Could you check a few things on this model? Use its own coordinates, in mm. Face numbers are marked on the shaded views. A direction names the side the tool comes from. Coordinates: 2 decimals unless noted, no trailing zeros. Order: outer loops, then holes, each group sorted by start corner. A loop starts at its lowest first (then second) coordinate and runs counter-clockwise, first axis right, second up. Notation, with made-up numbers: (-10.75, 68.25) -> (35.25, 68.25) arc R21 cw to (35.25, 94.25) -> close; hole circle Ø4 at (10, 0). An arc over 180 degrees is marked (long way). Put each result on its own line as item: value. Start each with the question number.
Q1. If we section it at B-B (z = -9.5): Please give me the cut outline in (x, y).
Q2. If we section it at C-C (x = -8): Please give me the cut outline in (y, z).
Q3. We'd pull the mould along Y, two halves only. Please class the marked faces 1, 2 and 3: +Y half, -Y half, draft (parallel to the pull), parting line (faces both ways), or undercut.
Q4. If we section it at D-D (y = -8): Please give me the cut outline in (x, z).
Q5. Please list where these lines run through material, in increasing order: line 1 along X through (y, z) = (4, -1); line 2 along Y through (x, z) = (22, -1.5); line 3 along Y through (x, z) = (-10, 0.75).
Q6. For the marked faces 4 and 5, which set-ups out of +Z, -Z, +X, -X, +Y, -Y let a thin tool reach every point of the face, with its end or its side?
Q7. If we section it at A-A (z = -3): Count the separate pieces of the cut face and the enclosed holes in it, and give its area (3 significant figures).
Q8. Will these pins go through, and if not, where does the flat tip stop? pin 1 (3.5 mm diameter, centred on x = -24.48, y = -11.95, fed in from +Z); pin 2 (1 mm diameter, centred on y = -2.5, z = -7.5, fed in from -X); pin 3 (4.5 mm diameter, centred on x = 22.12, y = -11.95, fed in from -Z); pin 4 (3 mm diameter, centred on x = 20, y = 3, fed in from -Z).
from build123d import *

# Parameters (mm, degrees)
CROQUIS2_R                = 2.4
CROQUIS2_R_2              = 1.45
SALIENTE_EXTRUIR2_DEPTH   = 12.3
SALIENTE_EXTRUIR2_2_DEPTH = 12.3
CROQUIS2_R_3              = 2.2627417
SALIENTE_EXTRUIR2_3_DEPTH = 12.3
CROQUIS2_R_4              = 1.304870774
SALIENTE_EXTRUIR2_4_DEPTH = 12.3
CROQUIS4_W                = 36.3
CROQUIS4_H                = 63.7
CROQUIS4_W_2              = 32.3
CROQUIS4_H_2              = 59.7
SALIENTE_EXTRUIR4_DEPTH   = 8.9
CROQUIS5_W                = 36.3
CROQUIS5_H                = 63.7
SALIENTE_EXTRUIR5_DEPTH   = 2
REDONDEO1_R               = 1
CROQUIS6_W                = 0.952491513
CROQUIS6_H                = 11.029714725
CORTAR_EXTRUIR1_DEPTH     = 1
REDONDEO2_R               = 1
CROQUIS7_R                = 1.45
CROQUIS7_R_2              = 1.304870774
CORTAR_EXTRUIR2_DEPTH     = 42.540563821
CROQUIS8_R                = 2.75
CORTAR_EXTRUIR3_DEPTH     = 1
CROQUIS9_R                = 3.250192478
CORTAR_EXTRUIR4_DEPTH     = 41.895212954
CROQUIS10_W               = 30.589236147
CROQUIS10_H               = 22.63620754
CROQUIS10_W_2             = 28.589236147
CROQUIS10_H_2             = 20.63620754
SALIENTE_EXTRUIR6_DEPTH   = 2.5


with BuildPart() as part:
    # Croquis2 → Saliente-Extruir2 (new body)
    with BuildSketch(Plane(origin=(-1.363345475, 4.236097797, 1), x_dir=(0, 1, 0), z_dir=(0, 0, 1))):
        with Locations(Location((-16.185020115, 23.120880637, 0), (0, 0, 270))):
            Circle(CROQUIS2_R)
        with Locations(Location((-16.185020115, 23.120880637, 0), (0, 0, 270))):
            Circle(CROQUIS2_R_2, mode=Mode.SUBTRACT)
    extrude(amount=-SALIENTE_EXTRUIR2_DEPTH)



with BuildPart() as body_2:
    # Croquis2 → Saliente-Extruir2 2 (new body)
    with BuildSketch(Plane(origin=(-1.363345475, 4.236097797, 1), x_dir=(0, 1, 0), z_dir=(0, 0, 1))):
        with Locations(Location((7.314979885, 23.120880637, 0), (0, 0, 270))):
            Circle(CROQUIS2_R)
        with Locations(Location((7.314979885, 23.120880637, 0), (0, 0, 270))):
            Circle(CROQUIS2_R_2, mode=Mode.SUBTRACT)
    extrude(amount=-SALIENTE_EXTRUIR2_2_DEPTH)


with BuildPart() as body_3:
    # Croquis2 → Saliente-Extruir2 3 (new body)
    with BuildSketch(Plane(origin=(-1.363345475, 4.236097797, 1), x_dir=(0, 1, 0), z_dir=(0, 0, 1))):
        with Locations(Location((7.314979885, -23.479119363, 0), (0, 0, 270))):
            Circle(CROQUIS2_R_3)
        with Locations(Location((7.314979885, -23.479119363, 0), (0, 0, 270))):
            Circle(CROQUIS2_R_2, mode=Mode.SUBTRACT)
    extrude(amount=-SALIENTE_EXTRUIR2_3_DEPTH)


with BuildPart() as body_4:
    # Croquis2 → Saliente-Extruir2 4 (new body)
    with BuildSketch(Plane(origin=(-1.363345475, 4.236097797, 1), x_dir=(0, 1, 0), z_dir=(0, 0, 1))):
        with Locations(Location((-16.185020115, -23.479119363, 0), (0, 0, 270))):
            Circle(CROQUIS2_R)
        with Locations(Location((-16.185020115, -23.479119363, 0), (0, 0, 270))):
            Circle(CROQUIS2_R_4, mode=Mode.SUBTRACT)
    extrude(amount=-SALIENTE_EXTRUIR2_4_DEPTH)


with BuildPart() as body_5:
    # Croquis4 → Saliente-Extruir4 (new body)
    with BuildSketch(Plane(origin=(-1.363345475, 4.236097797, 1), x_dir=(0, 1, 0), z_dir=(0, 0, 1))):
        with Locations((-4.435020115, -3.929119363)):
            Rectangle(CROQUIS4_W, CROQUIS4_H)
        with Locations((-4.435020115, -3.929119363)):
            Rectangle(CROQUIS4_W_2, CROQUIS4_H_2, mode=Mode.SUBTRACT)
    extrude(amount=-SALIENTE_EXTRUIR4_DEPTH)


with BuildPart() as part_1:
    add(part.part)

    add(body_2.part)  # Saliente-Extruir5 merges body 2

    add(body_3.part)  # Saliente-Extruir5 merges body 3

    add(body_4.part)  # Saliente-Extruir5 merges body 4

    add(body_5.part)  # Saliente-Extruir5 merges body 5
    # Croquis5 → Saliente-Extruir5 (add)
    with BuildSketch(Plane(origin=(-1.363345475, 4.236097797, 1), x_dir=(0, 1, 0), z_dir=(0, 0, 1))):
        with Locations((-4.435020115, -3.929119363)):
            Rectangle(CROQUIS5_W, CROQUIS5_H)
    extrude(amount=SALIENTE_EXTRUIR5_DEPTH)

    # Redondeo1
    redondeo1_edges = [part_1.edges().sort_by_distance(p)[0] for p in [
        (-29.284226112, -18.348922317, -2.45),
        (34.415773888, -18.348922317, -2.45),
        (34.415773888, 17.951077683, -2.45),
        (-29.284226112, 17.951077683, -2.45),
        (2.565773888, -18.348922317, 3),
        (34.415773888, -0.198922317, 3),
        (2.565773888, 17.951077683, 3),
        (-29.284226112, -0.198922317, 3),
    ]]
    fillet(redondeo1_edges, radius=REDONDEO1_R)

    # Croquis6 → Cortar-Extruir1 (cut)
    with BuildSketch(Plane.ZY.offset(29.284226112)):
        with Locations((-7.423754244, -0.221239115)):
            Rectangle(CROQUIS6_W, CROQUIS6_H)
    extrude(amount=-CORTAR_EXTRUIR1_DEPTH, mode=Mode.SUBTRACT)

    # Redondeo2
    redondeo2_edges = [part_1.edges().sort_by_distance(p)[0] for p in [
        (-29.284226112, -5.736096478, -7.423754243),
        (-29.284226112, 5.293618247, -7.423754243),
        (-29.284226112, -0.221239116, -6.947508487),
    ]]
    fillet(redondeo2_edges, radius=REDONDEO2_R - 0.0001)  # a hair under: the kernel refuses the full size

    # Croquis7 → Cortar-Extruir2 (cut, through all)
    with BuildSketch(Plane(origin=(0, 0, -11.3), x_dir=(-1, 0, 0), z_dir=(0, 0, -1))):
        with Locations(Location((24.484226112, 11.551077683, 0), (0, 0, 180))):
            Circle(CROQUIS7_R)
        with Locations(Location((24.484226112, -11.948922317, 0), (0, 0, 180))):
            Circle(CROQUIS7_R)
        with Locations(Location((-22.115773888, -11.948922317, 0), (0, 0, 180))):
            Circle(CROQUIS7_R_2)
        with Locations(Location((-22.115773888, 11.551077683, 0), (0, 0, 90))):
            Circle(CROQUIS7_R)
    extrude(amount=-CORTAR_EXTRUIR2_DEPTH, mode=Mode.SUBTRACT)

    # Croquis8 → Cortar-Extruir3 (cut)
    with BuildSketch(Plane.XY.offset(3)):
        with Locations((-24.484226112, -11.948922317)):
            Circle(CROQUIS8_R)
        with Locations((-24.484226112, 11.551077683)):
            Circle(CROQUIS8_R)
        with Locations((22.115773888, -11.948922317)):
            Circle(CROQUIS8_R)
        with Locations((22.115773888, 11.551077683)):
            Circle(CROQUIS8_R)
    extrude(amount=-CORTAR_EXTRUIR3_DEPTH, mode=Mode.SUBTRACT)

    # Croquis9 → Cortar-Extruir4 (cut, through all)
    with BuildSketch(Plane(origin=(0, 0, 1), x_dir=(-1, 0, 0), z_dir=(0, 0, -1))):
        with Locations((-27.415773888, 0.451077683)):
            Circle(CROQUIS9_R)
    extrude(amount=-CORTAR_EXTRUIR4_DEPTH, mode=Mode.SUBTRACT)

    # Croquis10 → Saliente-Extruir6 (add)
    with BuildSketch(Plane(origin=(0, 0, 1), x_dir=(-1, 0, 0), z_dir=(0, 0, -1))):
        with Locations((0.23483353, -0.007358301)):
            Rectangle(CROQUIS10_W, CROQUIS10_H)
        with Locations((0.234833529, -0.007358301)):
            Rectangle(CROQUIS10_W_2, CROQUIS10_H_2, mode=Mode.SUBTRACT)
    extrude(amount=SALIENTE_EXTRUIR6_DEPTH)


solid = part_1.part
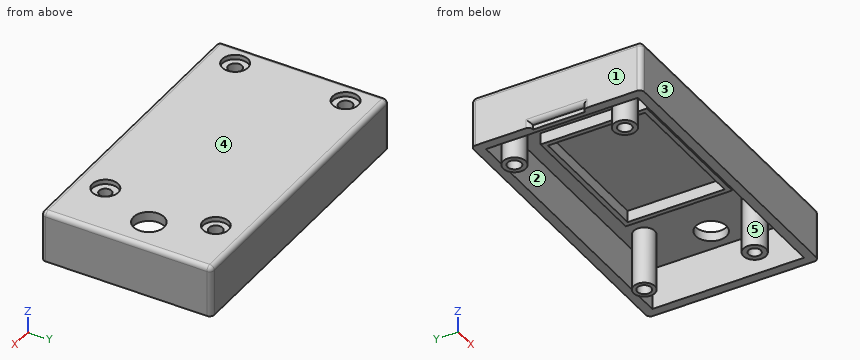
The answers:
1. outline: circle Ø4.8 at (-24.48, -11.95); circle Ø4.8 at (-24.48, 11.55); circle Ø4.8 at (22.12, -11.95); circle Ø4.53 at (22.12, 11.55); hole circle Ø2.9 at (-24.48, -11.95); hole circle Ø2.9 at (-24.48, 11.55); hole circle Ø2.9 at (22.12, 11.55); hole circle Ø2.61 at (22.12, -11.95)
2. outline: (-18.35, -7.9) -> (-16.35, -7.9) -> (-16.35, 1) -> (-11.33, 1) -> (-11.33, -1.5) -> (-10.33, -1.5) -> (-10.33, 1) -> (10.31, 1) -> (10.31, -1.5) -> (11.31, -1.5) -> (11.31, 1) -> (15.95, 1) -> (15.95, -7.9) -> (17.95, -7.9) -> (17.95, 2) arc R1 ccw to (16.95, 3) -> (-17.35, 3) arc R1 ccw to (-18.35, 2) -> close
3. face 1: draft
3. face 2: undercut
3. face 3: -Y half
4. outline: (-29.28, -7.9) -> (-27.28, -7.9) -> (-27.28, 1) -> (-15.53, 1) -> (-15.53, -1.5) -> (-14.53, -1.5) -> (-14.53, 1) -> (14.06, 1) -> (14.06, -1.5) -> (15.06, -1.5) -> (15.06, 1) -> (32.42, 1) -> (32.42, -7.9) -> (34.42, -7.9) -> (34.42, 2) arc R1 ccw to (33.42, 3) -> (-28.28, 3) arc R1 ccw to (-29.28, 2) -> close
5. line 1: -29.28 to -27.28, -15.53 to -14.53, 14.06 to 15.06, 32.42 to 34.42
5. line 2: -18.35 to -16.35, -14.35 to -13.25, -10.65 to -9.55, 9.29 to 10.11, 13 to 13.81, 15.95 to 17.95
5. line 3: -18.35 to -16.35, -11.33 to -10.33, 10.31 to 11.31, 15.95 to 17.95
6. face 4: +Z, +X, -X, +Y, -Y
6. face 5: -Z
7. separate pieces: 5
7. enclosed holes: 5
7. area: 428 mm^2
8. pin 1: z = 2
8. pin 2: x = -28.28
8. pin 3: z = -11.3
8. pin 4: z = 1
